Design review of the part built by this model. Coordinates are the model's own, in mm. A direction names the side the tool comes from. Round coordinates to 2 decimals unless told otherwise and drop trailing zeros. Loops run counter-clockwise (first coordinate to the right, second up) from the corner with the lowest first, then second, coordinate; pieces in that order, holes last. Notation, with made-up numbers: (39, 76) - (65, 76) arc R18 cw to (65, 103) - close; hole circle Ø9 at (-40, 4). An arc over 180 degrees is marked (long way). One line per question, with ' | ' between items. Start each with the question number.
from build123d import *

# Parameters (mm, degrees)
F0_W     = 41
F0_H     = 60
F1_DEPTH = 20
F2_W     = 37
F2_H     = 56
F3_DEPTH = 18
F5_W     = 6
F5_H     = 1.076952
F6_DEPTH = 2
F7_R     = 1.5
F8_DEPTH = 2


with BuildPart() as f1:
    # F0 (on Top) → F1 (new body)
    with BuildSketch(Plane.XY):
        Rectangle(F0_W, F0_H)
    extrude(amount=F1_DEPTH)

    # F2 (on face) → F3 (cut)
    with BuildSketch(Plane.XY.offset(20)):
        Rectangle(F2_W, F2_H)
    extrude(amount=-F3_DEPTH, mode=Mode.SUBTRACT)

    # F5 (on face) → F6 (cut)
    with BuildSketch(Plane.XZ.offset(-28)):
        with Locations((-11.5, 20.538476)):
            Rectangle(F5_W, F5_H)
    extrude(amount=-F6_DEPTH, mode=Mode.SUBTRACT)

    # F7 (on face) → F8 (cut)
    with BuildSketch(Plane.XY.offset(2)):
        with Locations((15.5, -25)):
            Circle(F7_R)
        with Locations((-15.5, -25)):
            Circle(F7_R)
    extrude(amount=-F8_DEPTH, mode=Mode.SUBTRACT)


solid = f1.part
1. Take a section at D-D, the plane y = -10. Give the boundary of the cut face in (x, z).
2. Clearance check with flat-ended pins moving along their axes: P1, Ø2, axis at x = 15.5, y = -12.5, coming from the -Z side; P2, Ø6, axis at x = 10, y = -9, coming from the +Z side. State where each tip first meets the part, or that it passes through.
3. To check wall thickness, follow line 1 along Y through (x, z) = (-15.5, 1.3); line 2 along X through (y, z) = (20.5, 3); line 3 along Y through (x, z) = (-2, 2.75). State the ranges of each line that lie inside material, in increasing order.
4. Machinability: for faces 1 (the face through (20.5, 0, 10)), 2 (the face through (0, 0, 2)), which of the approach directions +Z, -Z, +X, -X, +Y, -Y give a long, thin tool a straight path to every point of the face, cutting with its end or side? Answer none if there is none.
5. Take a section at A-A, the plane z = 4.5. Give the boundary of the cut face in (x, y), then the cut area to 3 significant figures.
6. Take a section at B-B, the plane x = -15.5. Give the boundary of the cut face in (y, z), then the cut area to 3 significant figures.
7. Take a section at C-C, the plane y = -25. Give the boundary of the cut face in (x, z), then the cut area to 3 significant figures.
Answer list:
1) outline: (-20.5, 0) - (20.5, 0) - (20.5, 20) - (18.5, 20) - (18.5, 2) - (-18.5, 2) - (-18.5, 20) - (-20.5, 20) - close
2) P1: stops at z = 0 | P2: stops at z = 2
3) line 1: y = -30 to -26.5, -23.5 to 30 | line 2: x = -20.5 to -18.5, 18.5 to 20.5 | line 3: y = -30 to -28, 28 to 30
4) face 1: +Z, -Z, +X, +Y, -Y | face 2: +Z
5) outline: (-20.5, -30) - (20.5, -30) - (20.5, 30) - (-20.5, 30) - close; hole (-18.5, -28) - (18.5, -28) - (18.5, 28) - (-18.5, 28) - close | area: 388 mm²
6) outline: (-30, 0) - (-26.5, 0) - (-26.5, 2) - (-28, 2) - (-28, 20) - (-30, 20) - close; (-23.5, 0) - (30, 0) - (30, 20) - (28, 20) - (28, 2) - (-23.5, 2) - close | area: 186 mm²
7) outline: (-20.5, 0) - (-17, 0) - (-17, 2) - (-18.5, 2) - (-18.5, 20) - (-20.5, 20) - close; (-14, 0) - (14, 0) - (14, 2) - (-14, 2) - close; (17, 0) - (20.5, 0) - (20.5, 20) - (18.5, 20) - (18.5, 2) - (17, 2) - close | area: 142 mm²
